Answer from the drawing. Dimensions are ordinates in mm from the lowest x, y and z of the part. Coordinates: 2 decimals unless noted, no trailing zeros. Write each loop counter-clockwise with the first axis right and the second up, starting at its lowest first coordinate (ties: lowest second). Pieces come first, ordered by that corner, then holes.
1) The part is cut by section D-D (x = 13.75). Determine the outline of the cut face in (y, z), then the cut area to 3 significant figures.
2) The part is cut by section A-A (x = 3). Determine the outline of the cut face in (y, z).
3) Determine the mould class of the marked faces 1, 2, 3 and 4 for opening direction X: +X half, -X half, draft (parallel to the pull), parting line (faces both ways), or undercut.
4) Each of these flat-tipped pins is pushed along its axis until it touches: pin 1 Ø0.9 at (y, z) = (3, 32) entering from -X; pin 2 Ø1.5 at (x, z) = (3, 18.5) entering from -Y; pin 3 Ø1 at (x, z) = (10.5, 29.5) entering from -Y. Where does it stop, or does it pass through?
5) Find the intervals of material crossed by line 1 (X direction, y = 17, z = 38.5); line 2 (Y direction, x = 9, z = 48.5), in increasing order.
6) The part is cut by section C-C (z = 17). Determine the outline of the cut face in (x, y).
7) The part is cut by section B-B (y = 16.25). Determine the outline of the cut face in (x, z).
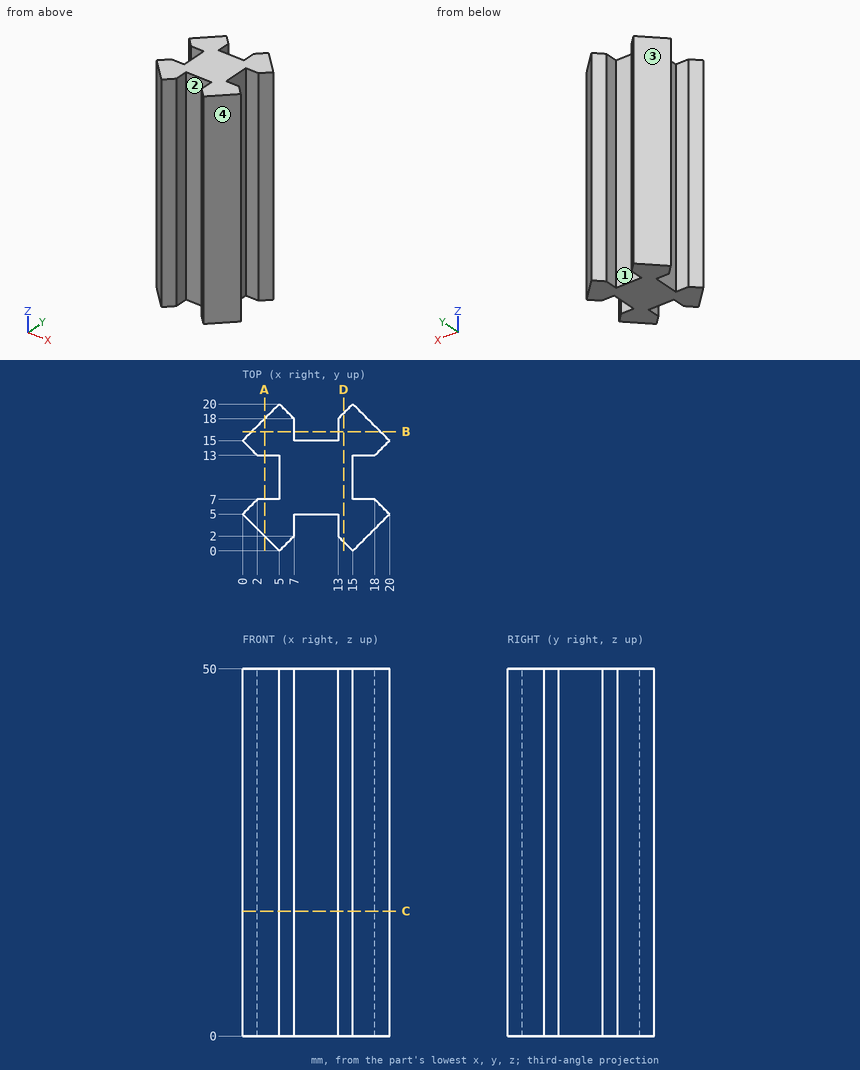
Reported:
1. outline: (1.25, 0) - (18.75, 0) - (18.75, 50) - (1.25, 50) - close
1. area: 875 mm2
2. outline: (2, 0) - (7, 0) - (7, 50) - (2, 50) - close; (13, 0) - (18, 0) - (18, 50) - (13, 50) - close
3. face 1: undercut
3. face 2: undercut
3. face 3: -X half
3. face 4: +X half
4. pin 1: stops at x = 1.55
4. pin 2: stops at y = 1.25
4. pin 3: stops at y = 5
5. line 1: x = 2 to 7, 13 to 18
5. line 2: y = 5 to 15
6. outline: (0, 5) - (5, 0) - (7, 2) - (7, 5) - (13, 5) - (13, 2) - (15, 0) - (20, 5) - (18, 7) - (15, 7) - (15, 13) - (18, 13) - (20, 15) - (15, 20) - (13, 18) - (13, 15) - (7, 15) - (7, 18) - (5, 20) - (0, 15) - (2, 13) - (5, 13) - (5, 7) - (2, 7) - close
7. outline: (1.25, 0) - (7, 0) - (7, 50) - (1.25, 50) - close; (13, 0) - (18.75, 0) - (18.75, 50) - (13, 50) - close
